Build history of the part. All positions in model axes, mm. Coordinates: 2 decimals unless noted, no trailing zeros. Loops run counter-clockwise (first coordinate to the right, second up) from the corner with the lowest first, then second, coordinate; pieces in that order, holes last.
(1) Wall check: L1, parallel to Y at x = 13, z = 0.9; L2, parallel to Y at x = -15, z = 1.25. Give the ranges that are in metal, low to high.
(2) Slice it at A-A (z = 1.7). Give the cut face in (x, y), and give its area (3 significant figures).
(3) Flat gauge pin, fed straight in: P1, Ø10, axis at x = 6.5, y = 8.5, coming from the -Z side. Where does the tip first touch, or does it go through?
(4) Slice it at B-B (y = -10). Give the cut face in (x, z), and give its area (3 significant figures).
from build123d import *

# Parameters (mm, degrees)
ESQUISSE1_W             = 36
ESQUISSE1_H             = 36
ESQUISSE1_W_2           = 30.1
ESQUISSE1_H_2           = 30.1
BOSS_EXTRU_1_DEPTH      = 2
ESQUISSE2_W             = 34
ESQUISSE2_H             = 34
ENL_V_MAT_EXTRU_1_DEPTH = 1


with BuildPart() as part:
    # Esquisse1 → Boss.-Extru.1 (new body)
    with BuildSketch(Plane.XY):
        Rectangle(ESQUISSE1_W, ESQUISSE1_H)
        Rectangle(ESQUISSE1_W_2, ESQUISSE1_H_2, mode=Mode.SUBTRACT)
    extrude(amount=BOSS_EXTRU_1_DEPTH)

    # Esquisse2 → Enlèv. mat.-Extru.1 (cut)
    with BuildSketch(Plane(origin=(0, 0, 0), x_dir=(-1, 0, 0), z_dir=(0, 0, -1))):
        Rectangle(ESQUISSE2_W, ESQUISSE2_H)
    extrude(amount=-ENL_V_MAT_EXTRU_1_DEPTH, mode=Mode.SUBTRACT)


solid = part.part
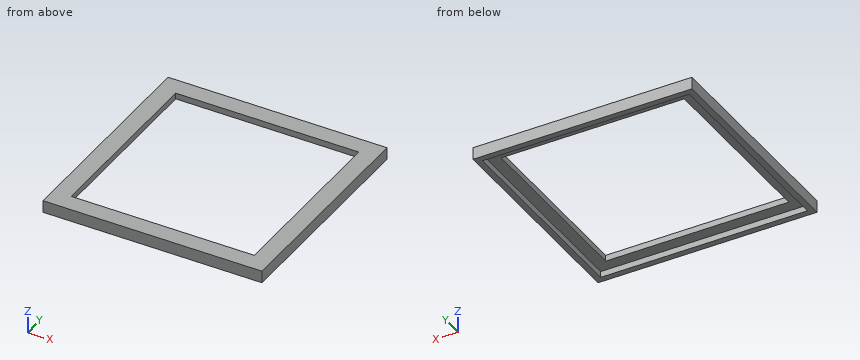
Response values:
1. L1: y = -18 to -17, 17 to 18
1. L2: y = -18 to -15.05, 15.05 to 18
2. outline: (-18, -18) - (18, -18) - (18, 18) - (-18, 18) - close; hole (-15.05, -15.05) - (15.05, -15.05) - (15.05, 15.05) - (-15.05, 15.05) - close
2. area: 390 mm2
3. P1: passes through
4. outline: (-18, 0) - (-17, 0) - (-17, 1) - (-15.05, 1) - (-15.05, 2) - (-18, 2) - close; (15.05, 1) - (17, 1) - (17, 0) - (18, 0) - (18, 2) - (15.05, 2) - close
4. area: 7.90 mm2
